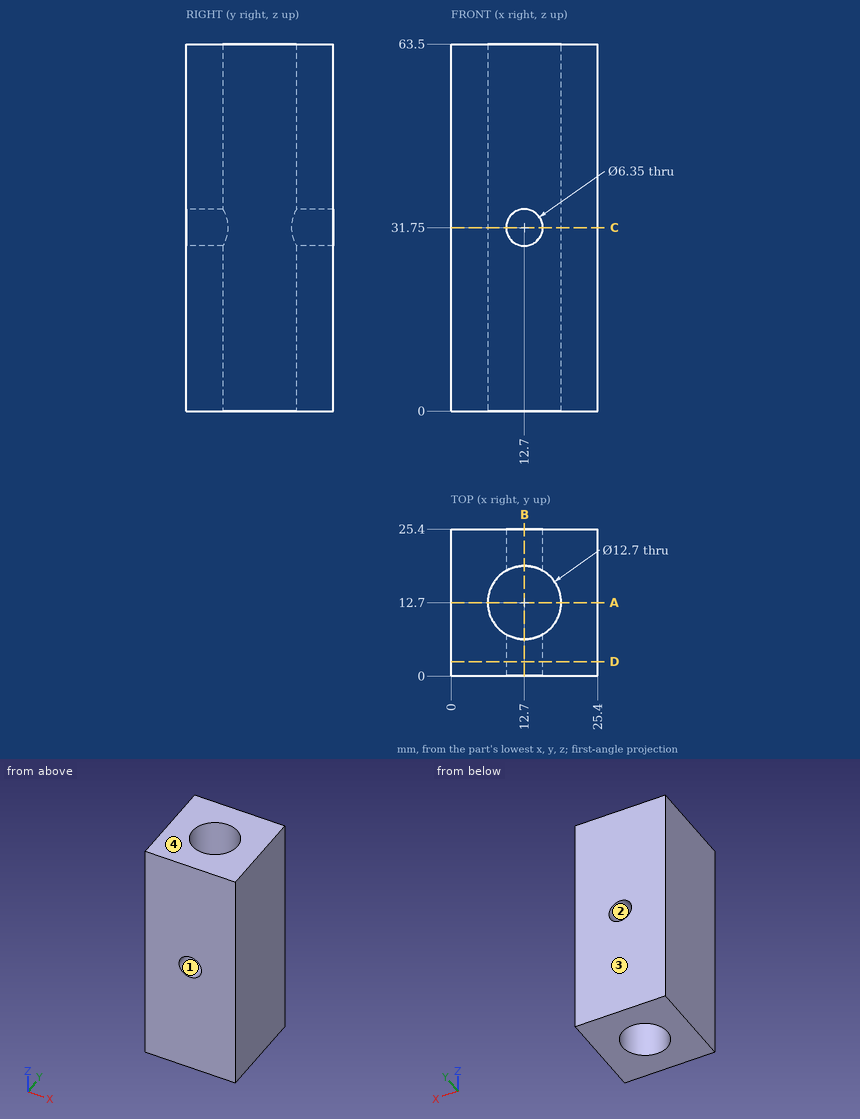
The drawing under review shows one solid part. Ordinate dimensions are in mm from its lowest x, y, z. Give positions to 0.01 mm unless a question says otherwise; leave off trailing zeros. Order: outer loops, then holes, each group sorted by start corner. A loop starts at its lowest first (then second) coordinate and runs counter-clockwise, first axis right, second up. Notation, with made-up numbers: M 78,40 L 136,40 A14 ccw 136,52 Z; hole C 29.25,43 d7. An arc over 180 degrees is marked long. Answer in a Markdown table with one row per item. Add a question column.
1. To check wall thickness, follow line 1 along Y through (x, z) = (12.7, 43.5); line 2 along Z through (x, y) = (12.7, 4.25) (3 decimals); line 3 along Y through (x, z) = (17.25, 9.5). State the ranges of each line that lie inside material, in increasing order.
2. For pin 1 Ø1.5 at (x, y) = (13.5, 16.5) entering from -Z, flat-tipped, find the tip position at first contact; note if it passes through.
3. Add section B-B on x = 12.7. State the section outline as (y, z) points (3 decimals).
4. Add section C-C on z = 31.75. State the section outline as (x, y) points (3 decimals).
5. Add section D-D on y = 2.5. State the section outline as (x, z) points (3 decimals), plus the area to 3 significant figures.
6. Add section A-A on y = 12.7. State the section outline as (x, z) points, plus the area to 3 significant figures.
7. Mouldability with a two-part tool opening along Z and no side actions: class the marked faces 1, 2, 3 and 4 as released by +Z, released by -Z, zero draft, split by the parting line, or undercut.
The answers:
| question | item | result |
|---|---|---|
| 1 | line 1 | 0 to 6.35, 19.05 to 25.4 |
| 1 | line 2 | 0 to 28.575, 34.925 to 63.5 |
| 1 | line 3 | 0 to 8.27, 17.13 to 25.4 |
| 2 | pin 1 | through |
| 3 | outline | M 0,0 L 6.35,0 L 6.35,28.575 L 0,28.575 Z; M 0,34.925 L 6.35,34.925 L 6.35,63.5 L 0,63.5 Z; M 19.05,0 L 25.4,0 L 25.4,28.575 L 19.05,28.575 Z; M 19.05,34.925 L 25.4,34.925 L 25.4,63.5 L 19.05,63.5 Z |
| 4 | outline | M 0,0 L 9.525,0 L 9.525,7.201 A6.35 cw 9.525,18.199 L 9.525,25.4 L 0,25.4 Z; M 15.875,0 L 25.4,0 L 25.4,25.4 L 15.875,25.4 L 15.875,18.199 A6.35 cw 15.875,7.201 Z |
| 5 | outline | M 0,0 L 25.4,0 L 25.4,63.5 L 0,63.5 Z; hole C 12.7,31.75 d6.35 |
| 5 | area | 1,580 mm2 |
| 6 | outline | M 0,0 L 6.35,0 L 6.35,63.5 L 0,63.5 Z; M 19.05,0 L 25.4,0 L 25.4,63.5 L 19.05,63.5 Z |
| 6 | area | 806 mm2 |
| 7 | face 1 | undercut |
| 7 | face 2 | undercut |
| 7 | face 3 | zero draft |
| 7 | face 4 | released by +Z |
